from build123d import *

# Parameters (mm, degrees)
Y_KSEKLIK_EKSTR_ZYON1_DEPTH = 120
RADYUS1_R                   = 20
KES_EKSTR_ZYON1_DEPTH       = 189.006716398
IZIM3_R                     = 7.5
KES_EKSTR_ZYON2_DEPTH       = 188.540730005


with BuildPart() as part:
    # Çizim1 → Yükseklik-Ekstrüzyon1 (new body)
    with BuildSketch(Plane.XY):
        Polygon((-23.340592334, 3.475609756), (46.659407666, 3.475609756), (46.659407666, -11.524390244), (-143.340592334, -11.524390244), (-143.340592334, 3.475609756), (-73.340592334, 3.475609756), (-73.340592334, 8.475609756), (-23.340592334, 8.475609756), align=None)
    extrude(amount=Y_KSEKLIK_EKSTR_ZYON1_DEPTH)

    # Radyus1
    radyus1_edges = [part.edges().sort_by_distance(p)[0] for p in [
        (46.659407666, -4.024390244, 0),
        (-143.340592334, -4.024390244, 0),
        (46.659407666, -4.024390244, 120),
        (-143.340592334, -4.024390244, 120),
    ]]
    fillet(radyus1_edges, radius=RADYUS1_R)

    # Çizim2 → Kes-Ekstrüzyon1 (cut, through all)
    with BuildSketch(Plane(origin=(0, 8.475609756, 0), x_dir=(1, 0, 0), z_dir=(0, 1, 0))):
        with BuildLine():
            Line((-38.340592334, -32.5), (-38.340592334, -87.5))
            ThreePointArc((-38.340592334, -87.5), (-48.340592334, -97.5), (-58.340592334, -87.5))
            Line((-58.340592334, -87.5), (-58.340592334, -32.5))
            ThreePointArc((-58.340592334, -32.5), (-48.340592334, -22.5), (-38.340592334, -32.5))
        make_face()
    extrude(amount=-KES_EKSTR_ZYON1_DEPTH, mode=Mode.SUBTRACT)

    # Çizim3 → Kes-Ekstrüzyon2 (cut, through all)
    with BuildSketch(Plane(origin=(0, 3.475609756, 0), x_dir=(1, 0, 0), z_dir=(0, 1, 0))):
        with Locations(Location((-123.340592334, -20, 0), (0, 0, 270))):
            Circle(IZIM3_R)
        with Locations(Location((-123.340592334, -100, 0), (0, 0, 270))):
            Circle(IZIM3_R)
        with Locations(Location((26.659407666, -100, 0), (0, 0, 90))):
            Circle(IZIM3_R)
        with Locations(Location((26.659407666, -20, 0), (0, 0, 90))):
            Circle(IZIM3_R)
    extrude(amount=-KES_EKSTR_ZYON2_DEPTH, mode=Mode.SUBTRACT)


solid = part.part
Model file for the job. Use its own axes, mm. A direction names the side the tool comes from. Coordinates: 2 decimals unless noted, no trailing zeros. Write each loop counter-clockwise with the first axis right and the second up, starting at its lowest first coordinate (ties: lowest second). Pieces come first, ordered by that corner, then holes. Notation, with made-up numbers: (-19, -5.75) -> (21, -5.75) arc R13 ccw to (21, 5.25) -> close; hole circle Ø2 at (50.25, 46). An arc over 180 degrees is marked (long way). One line per item, written item: value. Start each with the question number.
1) Slice it at D-D on x = -79.5. Write the cut outline in (y, z).
2) Flat gauge pins, fed straight in: pin 1 Ø1.5 at (y, z) = (7, 40.5) entering from -X; pin 2 Ø1.5 at (y, z) = (7, 84) entering from +X; pin 3 Ø1 at (x, z) = (-117.5, 16.5) entering from +Y (3 decimals); pin 4 Ø10 at (x, z) = (-104.5, 87.5) entering from +Y. Where does each tip first touch, or does it go through?
3) Pull direction X, two halves, no side cores. Call faces 1 (the face through (33.313, -3.919, 96.539)), 2 (the face through (-73.341, 6, 59)), 3 (the face through (11, 3.476, 59)), 4 (the face through (-130.66, -3.92, 18.37)): +X half, -X half, draft (parallel to the pull), parting line (faces both ways), or undercut.
4) Slice it at C-C on x = 22. Write the cut outline in (y, z).
5) Which spindle directions (+Z, -Z, +X, -X, +Y, -Y) get a long thin tool onto all of the face, cutting with end or side? Do faces 5 (the face through (-47, -4, 120)), 6 (the face through (-109, 3.476, 59)), 7 (the face through (-23.341, 6, 59)), 8 (the face through (-143.341, -4, 59)), 9 (the face through (-48.56, -1.384, 22.502)). Say none if no direction does.
6) Probe probe 1 along X at (y, z) = (-2.75, 100); probe 2 along X at (y, z) = (-3.75, 69.5); probe 3 along Z at (x, y) = (31.5, -8.25). List the from-to ranges inside material, lowest first.
7) Slice it at B-B on y = -9.5. Write the cut outline in (x, z).
8) Slice it at A-A on z = 61. Write the cut outline in (x, y).
Answers follow:
1. outline: (-11.52, 0) -> (3.48, 0) -> (3.48, 120) -> (-11.52, 120) -> close
2. pin 1: x = -73.34
2. pin 2: x = -23.34
2. pin 3: through
2. pin 4: y = 3.48
3. face 1: undercut
3. face 2: -X half
3. face 3: draft
3. face 4: undercut
4. outline: (-11.52, 0) -> (3.48, 0) -> (3.48, 14.12) -> (-11.52, 14.12) -> close; (-11.52, 25.88) -> (3.48, 25.88) -> (3.48, 94.12) -> (-11.52, 94.12) -> close; (-11.52, 105.88) -> (3.48, 105.88) -> (3.48, 120) -> (-11.52, 120) -> close
5. face 5: +Z, +X, -X, +Y, -Y
5. face 6: +Z, -Z, -X, +Y
5. face 7: +Z, -Z, +X, +Y
5. face 8: +Z, -Z, -X, +Y, -Y
5. face 9: +Y, -Y
6. probe 1: -143.34 to -130.84, -115.84 to 19.16, 34.16 to 46.66
6. probe 2: -143.34 to -58.34, -38.34 to 46.66
6. probe 3: 0.59 to 14.27, 25.73 to 94.27, 105.73 to 119.41
7. outline: (-143.34, 20) arc R20 ccw to (-123.34, 0) -> (26.66, 0) arc R20 ccw to (46.66, 20) -> (46.66, 100) arc R20 ccw to (26.66, 120) -> (-123.34, 120) arc R20 ccw to (-143.34, 100) -> close; hole circle Ø15 at (-123.34, 20); hole circle Ø15 at (-123.34, 100); hole (-58.34, 32.5) arc R10 ccw to (-38.34, 32.5) -> (-38.34, 87.5) arc R10 ccw to (-58.34, 87.5) -> close; hole circle Ø15 at (26.66, 20); hole circle Ø15 at (26.66, 100)
8. outline: (-143.34, -11.52) -> (-58.34, -11.52) -> (-58.34, 8.48) -> (-73.34, 8.48) -> (-73.34, 3.48) -> (-143.34, 3.48) -> close; (-38.34, -11.52) -> (46.66, -11.52) -> (46.66, 3.48) -> (-23.34, 3.48) -> (-23.34, 8.48) -> (-38.34, 8.48) -> close
